```python
from build123d import *

# Parameters (mm, degrees)
CROQUIS1_W              = 170
CROQUIS1_H              = 140
SALIENTE_EXTRUIR1_DEPTH = 20
CROQUIS2_W              = 170
CROQUIS2_H              = 140
CROQUIS2_W_2            = 156
CROQUIS2_H_2            = 126
CORTAR_EXTRUIR1_DEPTH   = 13
CROQUIS3_W              = 150
CROQUIS3_H              = 120
CORTAR_EXTRUIR2_DEPTH   = 18
CROQUIS4_R              = 1
CROQUIS4_W              = 28
CROQUIS4_H              = 29
CROQUIS4_W_2            = 19
CROQUIS4_H_2            = 32
CORTAR_EXTRUIR3_DEPTH   = 18
REDONDEO1_R             = 3


with BuildPart() as part:
    # Croquis1 → Saliente-Extruir1 (new body)
    with BuildSketch(Plane.XY):
        Rectangle(CROQUIS1_W, CROQUIS1_H)
    extrude(amount=SALIENTE_EXTRUIR1_DEPTH)

    # Croquis2 → Cortar-Extruir1 (cut)
    with BuildSketch(Plane(origin=(0, 0, 0), x_dir=(-1, 0, 0), z_dir=(0, 0, -1))):
        Rectangle(CROQUIS2_W, CROQUIS2_H)
        Rectangle(CROQUIS2_W_2, CROQUIS2_H_2, mode=Mode.SUBTRACT)
    extrude(amount=-CORTAR_EXTRUIR1_DEPTH, mode=Mode.SUBTRACT)

    # Croquis3 → Cortar-Extruir2 (cut)
    with BuildSketch(Plane(origin=(0, 0, 0), x_dir=(-1, 0, 0), z_dir=(0, 0, -1))):
        Rectangle(CROQUIS3_W, CROQUIS3_H)
    extrude(amount=-CORTAR_EXTRUIR2_DEPTH, mode=Mode.SUBTRACT)

    # Croquis4 → Cortar-Extruir3 (cut)
    with BuildSketch(Plane(origin=(0, 0, 18), x_dir=(-1, 0, 0), z_dir=(0, 0, -1))):
        with Locations((-46.5, -14)):
            Circle(CROQUIS4_R)
        with Locations((-46.5, 14)):
            Circle(CROQUIS4_R)
        with Locations((-70.5, -14)):
            Circle(CROQUIS4_R)
        with Locations((-70.5, 14)):
            Circle(CROQUIS4_R)
        with Locations((50, -34)):
            Rectangle(CROQUIS4_W, CROQUIS4_H)
        with Locations((50, 0)):
            Rectangle(CROQUIS4_W, CROQUIS4_H)
        with Locations((50, 34)):
            Rectangle(CROQUIS4_W, CROQUIS4_H)
        with Locations((14.5, 0)):
            Rectangle(CROQUIS4_W, CROQUIS4_H)
        with Locations((14.5, -34)):
            Rectangle(CROQUIS4_W, CROQUIS4_H)
        with Locations((-21, -34)):
            Rectangle(CROQUIS4_W, CROQUIS4_H)
        with Locations((14.5, 34)):
            Rectangle(CROQUIS4_W, CROQUIS4_H)
        with Locations((-21, 0)):
            Rectangle(CROQUIS4_W, CROQUIS4_H)
        with Locations((-21, 34)):
            Rectangle(CROQUIS4_W, CROQUIS4_H)
        with Locations((-58.5, 0)):
            Rectangle(CROQUIS4_W_2, CROQUIS4_H_2)
    extrude(amount=-CORTAR_EXTRUIR3_DEPTH, mode=Mode.SUBTRACT)

    # Redondeo1
    redondeo1_edges = [part.edges().sort_by_distance(p)[0] for p in [
        (-85, 0, 20),
        (0, -70, 20),
        (85, 0, 20),
        (0, 70, 20),
    ]]
    fillet(redondeo1_edges, radius=REDONDEO1_R)


solid = part.part
```
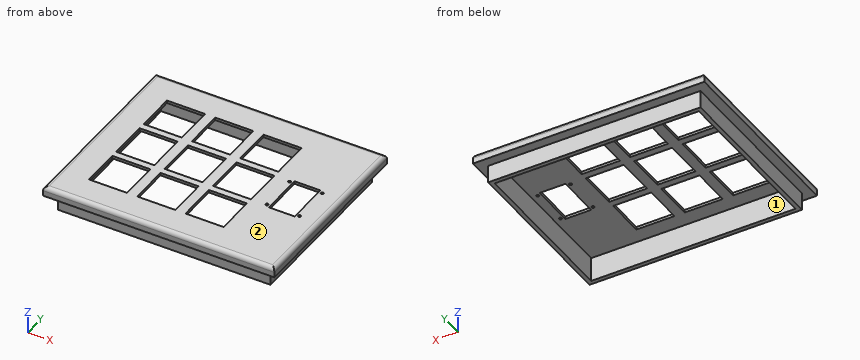
The model under review builds one solid part; all positions refer to its coordinate system, in mm. Face numbers are marked on the shaded views. Round coordinates to 2 decimals unless told otherwise and drop trailing zeros. Write each loop counter-clockwise with the first axis right and the second up, starting at its lowest first coordinate (ties: lowest second). Pieces come first, ordered by that corner, then holes. Notation, with made-up numbers: (-36, 45.25) - (1, 45.25) arc R15 ccw to (1, 74.25) - close; hole circle Ø11 at (70, -17.5). An arc over 180 degrees is marked (long way). Answer as CSV lines item,"result". Start each with the question number.
(1) We need section C-C on y = 40.5. State the section outline as (x, z) points.
(2) Draft analysis for pull direction Y (two halves, no side actions). For the marked faces 1 and 2, state which applies: pulls with the +Y half, pulls with the -Y half, needs draft (parallel to the pull), parting line crosses it, or undercut.
(3) We need section A-A on x = 52. State the section outline as (y, z) points, plus the area to 3 significant figures.
(4) To check wall thickness, follow line 1 (Y direction, x = -47.5, z = 2); line 2 (Y direction, x = 40.5, z = 14.5); line 3 (X direction, y = 50, z = 7.5). State the ranges of each line that lie inside material, in increasing order.
(5) We need section D-D on z = 9.5. State the section outline as (x, y) points, plus the area to 3 significant figures.
(6) We need section B-B on y = 3. Give the number of separate pieces and of enclosed holes in the cut face, plus the area to 3 significant figures.
(7) For pin 1 Ø1 at (x, z) = (-56.5, 19.5) entering from +Y; pin 2 Ø1 at (y, z) = (1, 19.5) entering from -X; pin 3 Ø1.5 at (x, z) = (-36, 3) entering from +Y, all flat-tipped, find the tip position at first contact; note any pin that passes through.
Worked answers:
1,outline,"(-85, 13) - (-78, 13) - (-78, 0) - (-75, 0) - (-75, 18) - (-64, 18) - (-64, 20) - (-82, 20) arc R3 ccw to (-85, 17) - close; (-36, 18) - (-28.5, 18) - (-28.5, 20) - (-36, 20) - close; (-0.5, 18) - (7, 18) - (7, 20) - (-0.5, 20) - close; (35, 18) - (75, 18) - (75, 0) - (78, 0) - (78, 13) - (85, 13) - (85, 17) arc R3 ccw to (82, 20) - (35, 20) - close"
2,face 1,"undercut"
2,face 2,"needs draft"
3,outline,"(-70, 13) - (-63, 13) - (-63, 0) - (-60, 0) - (-60, 18) - (-16, 18) - (-16, 20) - (-67, 20) arc R3 ccw to (-70, 17) - close; (16, 18) - (60, 18) - (60, 0) - (63, 0) - (63, 13) - (70, 13) - (70, 17) arc R3 ccw to (67, 20) - (16, 20) - close"
3,area,"390 mm²"
4,line 1,"-63 to -60, 60 to 63"
4,line 2,"-70 to -60, 60 to 70"
4,line 3,"-78 to -75, 75 to 78"
5,outline,"(-78, -63) - (78, -63) - (78, 63) - (-78, 63) - close; hole (-75, -60) - (75, -60) - (75, 60) - (-75, 60) - close"
5,area,"1,660 mm²"
6,separate pieces,"5"
6,enclosed holes,"0"
6,area,"308 mm²"
7,pin 1,"y = 69.24"
7,pin 2,"x = -84.24"
7,pin 3,"y = 63"
